from build123d import *

# Parameters (mm, degrees)
SKETCH1_R           = 31.75
SKETCH1_R_2         = 28.575
BOSS_EXTRUDE1_DEPTH = 508
SKETCH3_R           = 3.175
CUT_EXTRUDE1_DEPTH  = 508
SKETCH7_R           = 3.175
CUT_EXTRUDE2_DEPTH  = 64.5000001


with BuildPart() as part:
    # Sketch1 → Boss-Extrude1 (new body)
    with BuildSketch(Plane(origin=(0, 0, 0), x_dir=(1, 0, 0), z_dir=(0, 1, 0))):
        Circle(SKETCH1_R)
        Circle(SKETCH1_R_2, mode=Mode.SUBTRACT)
    extrude(amount=-BOSS_EXTRUDE1_DEPTH)

    # Sketch3 → Cut-Extrude1 (cut)
    with BuildSketch(Plane.XY.offset(31.75)):
        with Locations((0, -19.05)):
            Circle(SKETCH3_R)
        with Locations((0, -152.4)):
            Circle(SKETCH3_R)
    extrude(amount=-CUT_EXTRUDE1_DEPTH, mode=Mode.SUBTRACT)

    # Sketch7 → Cut-Extrude2 (cut, through all)
    with BuildSketch(Plane(origin=(31.75, 0, 0), x_dir=(0, 0, -1), z_dir=(1, 0, 0))):
        with Locations((0, -482.6)):
            Circle(SKETCH7_R)
    extrude(amount=-CUT_EXTRUDE2_DEPTH, mode=Mode.SUBTRACT)


solid = part.part
Could you check a few things on this model? Use its own coordinates, in mm. Coordinates: 2 decimals unless noted, no trailing zeros. Order: outer loops, then holes, each group sorted by start corner. A loop starts at its lowest first (then second) coordinate and runs counter-clockwise, first axis right, second up. Notation, with made-up numbers: (-32.75, 24) - (-17.75, 24) arc R30 ccw to (-17.75, 49) - close; hole circle Ø10 at (61, 30.25). An arc over 180 degrees is marked (long way). Answer in a Markdown table with one row per item. Add a question column.
(1) If we section it at B-B, the plane z = -13: Please give me the cut outline in (x, y), then the cut area to 3 significant figures.
(2) If we mould it in two halves opening along Z, with no side actions, what happens to faces 1 (the face through (-28.4, 0, -4.9)), 2 (the face through (-6.883, -250.444, 30.995)), 3 (the face through (-28.547, -250.444, -1.256))? For each: released by +Z, released by -Z, zero draft, split by the parting line, or undercut.
(3) Will these pins go through, and if not, where does the flat tip stop? pin 1 (12 mm diameter, centred on y = -204, z = -22.5, fed in from +X); pin 2 (2 mm diameter, centred on y = -123, z = -19, fed in from +X); pin 3 (5 mm diameter, centred on x = -17, y = -376.5, fed in from +Z).
(4) I need wall thicknesses on L1, parallel to Y at x = 0, z = -29 (3 decimals); L2, parallel to X at y = -311.5, z = -1.5; L3, parallel to Y at x = -29.3, z = 0 (3 decimals). Which ranges of each line are inside material? Lowest first, please.
(5) If we section it at A-A, the plane x = -19: Please give me the cut outline in (y, z).
Results are:
| question | item | result |
|---|---|---|
| 1 | outline | (-28.97, -508) - (-25.45, -508) - (-25.45, 0) - (-28.97, 0) - close; (25.45, -508) - (28.97, -508) - (28.97, 0) - (25.45, 0) - close |
| 1 | area | 3,580 mm2 |
| 2 | face 1 | zero draft |
| 2 | face 2 | split by the parting line |
| 2 | face 3 | undercut |
| 3 | pin 1 | stops at x = 27.13 |
| 3 | pin 2 | stops at x = 26.15 |
| 3 | pin 3 | stops at z = 28.25 |
| 4 | L1 | y = -508 to -155.575, -149.225 to -22.225, -15.875 to 0 |
| 4 | L2 | x = -31.71 to -28.54, 28.54 to 31.71 |
| 4 | L3 | y = -508 to -485.775, -479.425 to 0 |
| 5 | outline | (-508, -25.44) - (0, -25.44) - (0, -21.34) - (-508, -21.34) - close; (-508, 21.34) - (0, 21.34) - (0, 25.44) - (-508, 25.44) - close |
